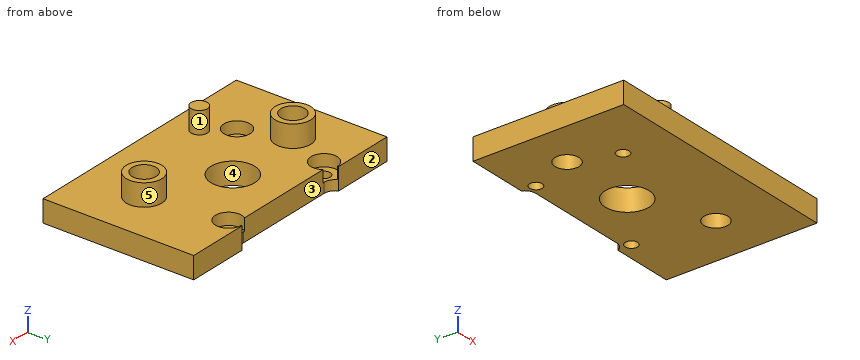
from build123d import *

# Parameters (mm, degrees)
SKETCH1_W                                        = 45
SKETCH1_H                                        = 27.5
BOSS_EXTRUDE1_DEPTH                              = 4
CUT_EXTRUDE1_DEPTH                               = 5
SKETCH3_W                                        = 3.25
SKETCH3_H                                        = 4
SKETCH4_W                                        = 1.5
SKETCH4_H                                        = 4
SKETCH5_W                                        = 3.25
SKETCH5_H                                        = 4
F_8_0_8_DIAMETER_HOLE1_D                         = 8
F_8_0_8_DIAMETER_HOLE1_DEPTH                     = 8
CBORE_FOR_M2_HEX_HEAD_MACHINE_SCREW1_D           = 2.26
CBORE_FOR_M2_HEX_HEAD_MACHINE_SCREW1_DEPTH       = 4
CBORE_FOR_M2_HEX_HEAD_MACHINE_SCREW1_CBORE_D     = 4.8
CBORE_FOR_M2_HEX_HEAD_MACHINE_SCREW1_CBORE_DEPTH = 2.18
TAPPED_HOLE_FOR_8_32_HELICOIL1_D                 = 4.3942
TAPPED_HOLE_FOR_8_32_HELICOIL1_DEPTH             = 13.335
TAPPED_HOLE_FOR_8_32_HELICOIL1_TIP               = 1.320150866


with BuildPart() as part:
    # Sketch1 → Boss-Extrude1 (new body)
    with BuildSketch(Plane.XY.offset(4)):
        with Locations((0, -3.25)):
            Rectangle(SKETCH1_W, SKETCH1_H)
    extrude(amount=-BOSS_EXTRUDE1_DEPTH)

    # Sketch2 → Cut-Extrude1 (cut, through all)
    with BuildSketch(Plane(origin=(0, 0, 0), x_dir=(-1, 0, 0), z_dir=(0, 0, -1))):
        with BuildLine():
            Line((-9.416969722, 9.3), (9.416969722, 9.3))
            ThreePointArc((9.416969722, 9.3), (10.512414837, 9.626679947), (11.25, 10.5))
            Line((11.25, 10.5), (-11.25, 10.5))
            ThreePointArc((-11.25, 10.5), (-10.512414837, 9.626679947), (-9.416969722, 9.3))
        make_face()
    extrude(amount=-CUT_EXTRUDE1_DEPTH, mode=Mode.SUBTRACT)

    # Sketch3 → Revolve1 (revolve)
    with BuildSketch(Plane(origin=(0, -6, 0), x_dir=(1, 0, 0), z_dir=(0, 1, 0))):
        with Locations((14.625, -6)):
            Rectangle(SKETCH3_W, SKETCH3_H)
    revolve(axis=Axis((13, -6, 4), (0, 0, 1)))

    # Sketch4 → Revolve2 (revolve)
    with BuildSketch(Plane(origin=(0, -12, 0), x_dir=(1, 0, 0), z_dir=(0, 1, 0))):
        with Locations((-6.75, -6)):
            Rectangle(SKETCH4_W, SKETCH4_H)
    revolve(axis=Axis((-7.5, -12, 4), (0, 0, 1)))

    # Sketch5 → Revolve3 (revolve)
    with BuildSketch(Plane(origin=(0, 0, 0), x_dir=(1, 0, 0), z_dir=(0, 1, 0))):
        with Locations((-12.375, -6)):
            Rectangle(SKETCH5_W, SKETCH5_H)
    revolve(axis=Axis((-14, 0, 4), (0, 0, 1)))

    # Ø8.0 (8) Diameter Hole1
    with Locations(Plane(origin=(0, 0, 0), x_dir=(-1, 0, 0), z_dir=(0, 0, -1))):
        with Locations((0, 0)):
            Hole(F_8_0_8_DIAMETER_HOLE1_D / 2, depth=F_8_0_8_DIAMETER_HOLE1_DEPTH)

    # CBORE for M2 Hex Head Machine Screw1
    with Locations(Plane.XY.offset(4)):
        with Locations((-11.113, -7.942), (-11.113, 7.938), (11.117, 7.938)):
            CounterBoreHole(CBORE_FOR_M2_HEX_HEAD_MACHINE_SCREW1_D / 2, CBORE_FOR_M2_HEX_HEAD_MACHINE_SCREW1_CBORE_D / 2, CBORE_FOR_M2_HEX_HEAD_MACHINE_SCREW1_CBORE_DEPTH, depth=CBORE_FOR_M2_HEX_HEAD_MACHINE_SCREW1_DEPTH)

    # Tapped Hole for #8-32 Helicoil1
    with Locations(Plane.XY.offset(8)):
        with Locations((-14, 0), (13, -6)):
            Hole(TAPPED_HOLE_FOR_8_32_HELICOIL1_D / 2, depth=TAPPED_HOLE_FOR_8_32_HELICOIL1_DEPTH)
            with Locations((0, 0, -(TAPPED_HOLE_FOR_8_32_HELICOIL1_DEPTH + TAPPED_HOLE_FOR_8_32_HELICOIL1_TIP / 2))):  # 118° drill point
                Cone(0, TAPPED_HOLE_FOR_8_32_HELICOIL1_D / 2, TAPPED_HOLE_FOR_8_32_HELICOIL1_TIP, mode=Mode.SUBTRACT)


solid = part.part
Model file for the job. Use its own axes, mm. Face numbers are marked on the shaded views. A direction names the side the tool comes from. Round coordinates to 2 decimals unless told otherwise and drop trailing zeros. Order: outer loops, then holes, each group sorted by start corner. A loop starts at its lowest first (then second) coordinate and runs counter-clockwise, first axis right, second up. Notation, with made-up numbers: M 76,36 L 123,36 A14 ccw 123,46 Z; hole C 4,-12 d6. An arc over 180 degrees is marked long. Write each question's results on one line, items separated by ' | '. Start each with the question number.
(1) Saw through at A-A, the plane z = 6. Give the cut face in (x, y), then the cut area to 3 significant figures.
(2) Probe probe 1 along Y at (x, z) = (-14, 2); probe 2 along X at (y, z) = (1.5, 2.5); probe 3 along Y at (x, z) = (13, 4.75). List the from-to ranges inside material, lowest first. Write a range as from..to.
(3) Which spindle directions (+Z, -Z, +X, -X, +Y, -Y) get a long thin tool onto all of the face, cutting with end or side? Do the marked faces 1 and 2. Say none if no direction does.
(4) Saw through at D-D, the plane y = -12. Give the cut face in (x, z), then the cut area to 3 significant figures.
(5) Two-plate mould, pull along Y, no slides. Class the marked faces 3, 4 and 5: pulls with the +Y half, pulls with the -Y half, needs draft (parallel to the pull), parting line crosses it, or undercut.
(6) Saw through at B-B, the plane y = 0. Give the cut face in (x, z).
(7) Saw through at C-C, the plane x = -14. Give the cut face in (y, z), then the cut area to 3 significant figures.
(8) Drop flat-ended pins along their axis: pin 1 (1.5 mm diameter, centred on y = -10, z = 6.5, fed in from -X); pin 2 (4 mm diameter, centred on x = -12, y = -8.5, fed in from +Z); pin 3 (1.5 mm diameter, centred on x = -12.5, z = 5.5, fed in from +Y). Give the stop position or say it passes through.
Established:
1) outline: C -14,0 d6.5; C -7.5,-12 d3; C 13,-6 d6.5; hole C -14,0 d4.39; hole C 13,-6 d4.39 | area: 43.1 mm^2
2) probe 1: y = -17..-2.2, 2.2..10.5 | probe 2: x = -22.5..-15.61, -12.39..-3.71, 3.71..22.5 | probe 3: y = -9.25..-8.2, -3.8..-2.75
3) face 1: +Z | face 2: +Z, -Z, +X, -X, +Y
4) outline: M -22.5,0 L 22.5,0 L 22.5,4 L -6,4 L -6,8 L -9,8 L -9,4 L -22.5,4 Z | area: 192 mm^2
5) face 3: pulls with the +Y half | face 4: undercut | face 5: parting line crosses it
6) outline: M -22.5,0 L -16.2,0 L -16.2,8 L -17.25,8 L -17.25,4 L -22.5,4 Z; M -11.8,0 L -4,0 L -4,4 L -10.75,4 L -10.75,8 L -11.8,8 Z; M 4,0 L 22.5,0 L 22.5,4 L 4,4 Z
7) outline: M -17,0 L -2.2,0 L -2.2,8 L -3.25,8 L -3.25,4 L -17,4 Z; M 2.2,0 L 10.5,0 L 10.5,4 L 3.25,4 L 3.25,8 L 2.2,8 Z | area: 101 mm^2
8) pin 1: stops at x = -8.33 | pin 2: stops at z = 4 | pin 3: stops at y = 3.16
